Check sheet for the modelled part. Datum: model origin and axes. Units: mm. A direction names the side the tool comes from. Give positions to 0.01 mm unless a question says otherwise; leave off trailing zeros. Order: outer loops, then holes, each group sorted by start corner. A loop starts at its lowest first (then second) coordinate and runs counter-clockwise, first axis right, second up. Notation, with made-up numbers: (-29.5, 52) -> (-23.5, 52) arc R20 cw to (-23.5, 64) -> close; hole circle Ø10 at (-27.5, -24.5). An arc over 180 degrees is marked (long way). Answer in a Markdown table with one row per item. Add a question column.
(1) Cross-section at C-C (x = 8.5). Record the cut outline in (y, z).
(2) Cross-section at D-D (z = -20.5). Record the cut outline in (x, y), then the cut area to 3 significant figures.
(3) Thickness scan on L1, parallel to Y at x = -14, z = -17; L2, parallel to X at y = -45.5, z = -17; L3, parallel to X at y = -62.5, z = -48. Record the ranges inside material, lowest first. Write a range as [from, to].
(4) Set-up check for faces 4 (the face through (16.258, -32.967, -38.419)), 5 (the face through (-5.326, -33, -55)), 6 (the face through (0, -1, -18.978)): record each of +Z, -Z, +X, -X, +Y, -Y from which the full face is reachable in a straight line by a thin tool's end or side.
(5) Go/stop test with flat-tipped pins: pin 1 (3 mm diameter, centred on y = -41, z = -54.5, fed in from +X); pin 2 (1.5 mm diameter, centred on x = 12, y = -31.5, fed in from -Z); pin 3 (4 mm diameter, centred on y = -20.5, z = -45, fed in from -X). Record where each tip stops, or that it passes through.
(6) Cross-section at A-A (y = -36.5). Record the cut outline in (x, z).
(7) Release check for a two-part mould opening along Z. For faces 1 (the face through (-16.57, -32.97, -37.99)), 2 (the face through (-1.25, -66, -17)), 3 (the face through (-6, -31, -55.978)) record: released by +Z, released by -Z, zero draft, split by the parting line, or undercut.
(8) Cross-section at B-B (z = -27.5). Record the cut outline in (x, y), then the cut area to 3 significant figures.
```python
from build123d import *

# Parameters (mm, degrees)
F1_DEPTH = 66.8
F2_T     = -2.5
F3_DEPTH = 25
F5_DEPTH = 25
F6_R     = 0.2
F8_DEPTH = 25
F9_R     = 0.2


with BuildPart() as f1:
    # F0 (on Front) → F1 (new body)
    with BuildSketch(Plane.XZ):
        Polygon((0, -55.9782199562), (0, 4.0217800438), (-30, 4.0217800438), (-30, -23.7439740449), (-6.6, -55.9782199562), align=None)
        Polygon((30, 4.0217800438), (0, 4.0217800438), (0, -55.9782199562), (6.6, -55.9782199562), (30, -23.7439740449), align=None)
    extrude(amount=F1_DEPTH)

    # F2
    f2_openings = [f1.faces().sort_by_distance(p)[0] for p in [
        (0, -33.4, 4.02178),
    ]]
    offset(amount=F2_T, openings=f2_openings)

    # F3 (cut): a face of the model
    f3_faces = [f1.faces().sort_by_distance(p)[0] for p in [
        (0, -33.4, -53.4782199562),
    ]]
    extrude(f3_faces, amount=-F3_DEPTH, mode=Mode.SUBTRACT)

    # F4 (on face) → F5 (cut)
    with BuildSketch(Plane.XZ.offset(66.8)):
        Polygon((-2.4, -8.6), (-2.4, -11.6), (-1.25, -11.6), (-1.25, -21.6), (0, -21.6), (0, -8.6), align=None)
        Polygon((2.4, -8.6), (0, -8.6), (0, -21.6), (1.25, -21.6), (1.25, -11.6), (2.4, -11.6), align=None)
    extrude(amount=-F5_DEPTH, mode=Mode.SUBTRACT)

    # F6
    f6_edges = [f1.edges().sort_by_distance(p)[0] for p in [
        (1.25, -65.55, -11.6),
        (-1.25, -65.55, -11.6),
        (0, -64.3, -8.6),
        (2.4, -64.3, -10.1),
        (1.825, -64.3, -11.6),
        (1.25, -64.3, -16.6),
        (-2.4, -64.3, -10.1),
        (-1.825, -64.3, -11.6),
        (0, -64.3, -21.6),
        (-1.25, -64.3, -16.6),
    ]]
    fillet(f6_edges, radius=F6_R)

    # F7 (on face) → F8 (cut)
    with BuildSketch(Plane(origin=(0, 0, 0), x_dir=(-1, 0, 0), z_dir=(0, 1, 0))):
        Polygon((1.5, -7.9782199562), (0, -7.9782199562), (-1.5, -7.9782199562), (-1.5, -18.9782199562), (0, -18.9782199562), (1.5, -18.9782199562), align=None)
    extrude(amount=-F8_DEPTH, mode=Mode.SUBTRACT)

    # F9
    f9_edges = [f1.edges().sort_by_distance(p)[0] for p in [
        (0, -2.5, -7.97822),
    ]]
    fillet(f9_edges, radius=F9_R)


solid = f1.part
```
Answer below:
| question | item | result |
|---|---|---|
| 1 | outline | (-66.8, -53.36) -> (0, -53.36) -> (0, 4.02) -> (-2.5, 4.02) -> (-2.5, -49.11) -> (-64.3, -49.11) -> (-64.3, 4.02) -> (-66.8, 4.02) -> close |
| 2 | outline | (-30, -66.8) -> (-1.25, -66.8) -> (-1.25, -64.5) arc R0.2 ccw to (-1.45, -64.3) -> (-27.5, -64.3) -> (-27.5, -2.5) -> (27.5, -2.5) -> (27.5, -64.3) -> (1.45, -64.3) arc R0.2 ccw to (1.25, -64.5) -> (1.25, -66.8) -> (30, -66.8) -> (30, 0) -> (-30, 0) -> close |
| 2 | area | 603 mm² |
| 3 | L1 | y = [-66.8, -64.3], [-2.5, 0] |
| 3 | L2 | x = [-30, -27.5], [27.5, 30] |
| 3 | L3 | x = [-12.39, -9.3], [9.3, 12.39] |
| 4 | face 4 | +Z |
| 4 | face 5 | +Z, -Z |
| 4 | face 6 | +Y |
| 5 | pin 1 | stops at x = 8.76 |
| 5 | pin 2 | stops at z = -49.57 |
| 5 | pin 3 | stops at x = -16.02 |
| 6 | outline | (-30, -23.74) -> (-6.6, -55.98) -> (-5.33, -55.98) -> (-5.33, -53.48) -> (-27.5, -22.93) -> (-27.5, 4.02) -> (-30, 4.02) -> close; (5.33, -55.98) -> (6.6, -55.98) -> (30, -23.74) -> (30, 4.02) -> (27.5, 4.02) -> (27.5, -22.93) -> (5.33, -53.48) -> close |
| 7 | face 1 | released by +Z |
| 7 | face 2 | undercut |
| 7 | face 3 | released by -Z |
| 8 | outline | (-27.27, -66.8) -> (27.27, -66.8) -> (27.27, 0) -> (-27.27, 0) -> close; hole (-24.18, -64.3) -> (24.18, -64.3) -> (24.18, -2.5) -> (-24.18, -2.5) -> close |
| 8 | area | 655 mm² |
